Geometry check sheet. Reference: the model listing, model coordinates, mm. A direction names the side the tool comes from. Give positions to 0.01 mm unless a question says otherwise; leave off trailing zeros. Order: outer loops, then holes, each group sorted by start corner. A loop starts at its lowest first (then second) coordinate and runs counter-clockwise, first axis right, second up. Notation, with made-up numbers: (74, 73) - (126, 73) arc R15 ccw to (126, 87) - close; hole circle Ø1 at (-27.75, 8.5). An arc over 180 degrees is marked (long way). Put each result on its own line as item: value. Start each with the question number.
Autodesk Inventor part; units mm, degrees
ref_plane "YZ Plane" through (0, 0, 0) normal (1, 0, 0) x (0, 1, 0)
ref_plane "XZ Plane" through (0, 0, 0) normal (0, 1, 0) x (-1, 0, 0)
ref_plane "XY Plane" through (0, 0, 0) normal (0, 0, 1) x (1, 0, 0)
sketch "Boceto1" plane through (0, 0, 0) normal (0, 1, 0) x (-1, 0, 0)
  circle A0 centre (14.1421, -14.1421) radius 3.5
  circle A1 centre (-14.1421, -14.1421) radius 3.5
  circle A2 centre (-14.1421, 14.1421) radius 3.5
  circle A3 centre (14.1421, 14.1421) radius 3.5
  circle A4 centre (0, 0) radius 25
  circle A5 centre (0, 0) radius 20
  dimension "d24" = 40
  dimension "d23" = 7
  dimension "d25" = 50
  dimension "d26" = 7
  dimension "d27" = 7
  dimension "d28" = 7
extrude "Extrusión1" add sketch "Boceto1" along normal blind 10 contours A0 A5 A1 A2 A3 | A4
sketch "Boceto2" plane through (0, 10, 0) normal (0, 1, 0) x (1, 0, 0)
  line L0 (0, 0) -> (3, 0)
  line L1 (3, 0) -> (3, 24.8193)
  circle A0 centre (0, 0) radius 25
  line L2 (0, 0) -> (-3, 0)
  line L3 (-3, 0) -> (-3, 24.8193)
  arc A1 (3, 24.8193) -> (-3, 24.8193) centre (0, 0) ccw
  dimension "d13" = 3
  dimension "d14" = 3
extrude "Extrusión2" add sketch "Boceto2" along normal blind 40 contours L2 L3 A0 L1 L0 picked at (-2, 8.2731)
fillet "Empalme1" radius 10 1 edges at (0, 50, 0)
fillet "Empalme2" radius 10 1 edges at (0, 50, -25)
fillet "Empalme3" radius 4 3 edges at (3, 10, -12.4097) (0, 10, 0) (-3, 10, -12.4097)
sketch "Boceto3" plane through (3, 50, -10) normal (1, 0, 0) x (0, 0, -1)
  line L0 (-10, -36) -> (-10, -10)
  line L1 (14.8193, -36) -> (14.8193, -10)
  circle A0 centre (2.4097, -10) radius 3
  point P0 (-10, -50)
extrude "Extrusión3" cut sketch "Boceto3" against normal blind 40
properties part number "Base"
Item 1: Cross-section at D-D (z = 1.5). Enter the section's corners in (x, y), and give its area (3 significant figures).
Item 2: Release check for a two-part mould opening along X. For faces 6 (the face through (4.203, 11.141, -10.611)), 7 (the face through (-0.1, 10.75, 1.67)), 8 (the face through (10.804, 4.93, -15.193)) record: +X half, -X half, draft (parallel to the pull), parting line (faces both ways), or undercut.
Item 3: Thickness scan on line 1 along Z through (x, y) = (17, 7.5); line 2 along Y through (x, z) = (0, 6.5); line 3 along X through (y, z) = (37, -7). Record the ranges inside material, lowest first.
Item 4: Cross-section at A-A (x = 0). Enter the section's corners in (y, z), and give its area (3 significant figures).
Item 5: Gauge pin test, flat ends, axial feed: pin 1 Ø20 at (y, z) = (40.5, -17) entering from -X; pin 2 Ø1.5 at (x, z) = (-2.5, 2.5) entering from +Y; pin 3 Ø2 at (y, z) = (43.5, -13.5) entering from +X. Record the tip position at first contact, or that the pin passes through.
Item 6: Cross-section at C-C (y = 38). Enter the section's corners in (x, z).
Item 7: Set-up check for faces 1 (the face through (0, 27, 0)), 2 (the face through (3, 32, -12)), 3 (the face through (12.53, 4.93, 17.25)), 4 (the face through (-3, 32, -12)), 5 (the face through (0, 10, 6)): record each of +Z, -Z, +X, -X, +Y, -Y from which the full face is reachable in a straight line by a thin tool's end or side.
Item 8: Cross-section at B-B (x = -13). Enter the section's corners in (y, z).
Recorded:
1. outline: (-24.95, 0) - (24.95, 0) - (24.95, 10) - (7, 10) arc R4 cw to (4.5, 10.88) - (-4.5, 10.88) arc R4 cw to (-7, 10) - (-24.95, 10) - close
1. area: 508 mm^2
2. face 6: +X half
2. face 7: draft
2. face 8: undercut
3. line 1: z = -18.33 to -16.16, -12.12 to 12.12, 16.16 to 18.33
3. line 2: y = 0 to 10
3. line 3: x = -3 to 3
4. outline: (0, -25) - (40, -25) arc R10 ccw to (50, -15) - (50, -10) arc R10 ccw to (40, 0) - (14, 0) arc R4 cw to (10, 4) - (10, 25) - (0, 25) - close; hole circle Ø6 at (40, -12.41)
4. area: 1,430 mm^2
5. pin 1: stops at x = -3
5. pin 2: stops at y = 10.69
5. pin 3: stops at x = 3
6. outline: (-3, -24.82) arc R25 ccw to (3, -24.82) - (3, -14.65) - (-3, -14.65) - close; (-3, -10.17) - (3, -10.17) - (3, 0) - (-3, 0) - close
7. face 1: +Z, +X, -X, +Y
7. face 2: +Z, -Z, +X, +Y
7. face 3: +Y, -Y
7. face 4: +Z, -Z, -X, +Y
7. face 5: +Z, +Y
8. outline: (0, -21.35) - (10, -21.35) - (10, -17.45) - (0, -17.45) - close; (0, -10.83) - (10, -10.83) - (10, 10.83) - (0, 10.83) - close; (0, 17.45) - (10, 17.45) - (10, 21.35) - (0, 21.35) - close
